```python
from build123d import *

# Parameters (mm, degrees)
BOSS_EXTRUDE1_DEPTH       = 276.125
SKETCH3_W                 = 268.125
SKETCH3_H                 = 78.2
CUT_EXTRUDE1_DEPTH        = 21
SKETCH4_W                 = 14
SKETCH4_H                 = 14.4
CUT_EXTRUDE2_DEPTH        = 4
FILLET1_R                 = 5
FILLET4_R                 = 3
FILLET5_R                 = 4
FILLET6_R                 = 4
SKETCH5_R                 = 2.5
BOSS_EXTRUDE2_DEPTH       = 5
FILLET7_R                 = 3
M2X0_4_TAPPED_HOLE4_D     = 1.6
M2X0_4_TAPPED_HOLE4_DEPTH = 3.719311505
M2X0_4_TAPPED_HOLE4_TIP   = 0.480688495
CUT_EXTRUDE3_DEPTH        = 2
FILLET8_R                 = 3
SKETCH10_R                = 5
CUT_EXTRUDE4_DEPTH        = 0.5


with BuildPart() as part:
    # Sketch1 → Boss-Extrude1 (new body)
    with BuildSketch(Plane(origin=(0, 0, 0), x_dir=(0, 0, -1), z_dir=(1, 0, 0))):
        Polygon((43.1, -11), (43.1, -18.54), (-43.1, -11), (-43.1, 11), (43.1, 11), align=None)
    extrude(amount=BOSS_EXTRUDE1_DEPTH)

    # Sketch3 → Cut-Extrude1 (cut)
    with BuildSketch(Plane(origin=(0, 11, 0), x_dir=(1, 0, 0), z_dir=(0, 1, 0))):
        with Locations((138.0625, 0)):
            Rectangle(SKETCH3_W, SKETCH3_H)
    extrude(amount=-CUT_EXTRUDE1_DEPTH, mode=Mode.SUBTRACT)

    # Sketch4 → Cut-Extrude2 (cut)
    with BuildSketch(Plane.XY.offset(-39.1)):
        with Locations((257.755, 3.8)):
            Rectangle(SKETCH4_W, SKETCH4_H)
    extrude(amount=-CUT_EXTRUDE2_DEPTH, mode=Mode.SUBTRACT)

    # Fillet1
    fillet1_edges = [part.edges().sort_by_distance(p)[0] for p in [
        (276.125, -3.77, -43.1),
        (276.125, 0, 43.1),
        (0, -3.77, -43.1),
        (0, 0, 43.1),
    ]]
    fillet(fillet1_edges, radius=FILLET1_R)

    # Fillet4
    fillet4_edges = [part.edges().sort_by_distance(p)[0] for p in [
        (272.125, 0.5, -39.1),
        (272.125, 0.5, 39.1),
        (4, 0.5, 39.1),
        (4, 0.5, -39.1),
    ]]
    fillet(fillet4_edges, radius=FILLET4_R)

    # Fillet5
    fillet5_edges = [part.edges().sort_by_distance(p)[0] for p in [
        (264.755, 11, -41.1),
        (264.755, -3.4, -41.1),
        (250.755, -3.4, -41.1),
        (250.755, 11, -41.1),
    ]]
    fillet(fillet5_edges, radius=FILLET5_R)

    # Fillet6
    fillet6_edges = [part.edges().sort_by_distance(p)[0] for p in [
        (274.660533906, 11, 41.635533906),
        (276.125, 11, 0),
        (274.660533906, 11, -41.635533906),
        (269.94, 11, -43.1),
        (265.926572875, 9.828427125, -43.1),
        (264.755, 3.8, -43.1),
        (263.583427125, -2.228427125, -43.1),
        (257.755, -3.4, -43.1),
        (251.926572875, -2.228427125, -43.1),
        (250.755, 3.8, -43.1),
        (249.583427125, 9.828427125, -43.1),
        (125.8775, 11, -43.1),
        (1.464466094, 11, -41.635533906),
        (0, 11, 0),
        (1.464466094, 11, 41.635533906),
        (138.0625, 11, 43.1),
    ]]
    fillet(fillet6_edges, radius=FILLET6_R - 0.0001)  # a hair under: the kernel refuses the full size

    # Sketch5 → Boss-Extrude2 (add)
    with BuildSketch(Plane(origin=(0, -10, 0), x_dir=(1, 0, 0), z_dir=(0, 1, 0))):
        with Locations(Location((240.4, 19.1, 0), (0, 0, 90))):
            Circle(SKETCH5_R)
        with Locations(Location((240.4, -19, 0), (0, 0, 90))):
            Circle(SKETCH5_R)
        with BuildLine():
            Line((9.8, 21.6), (4, 21.6))
            Line((4, 21.6), (4, 16.6))
            Line((4, 16.6), (9.8, 16.6))
            ThreePointArc((9.8, 16.6), (12.3, 19.1), (9.8, 21.6))
        make_face()
        with BuildLine():
            Line((9.8, -16.5), (4, -16.5))
            Line((4, -16.5), (4, -21.5))
            Line((4, -21.5), (9.8, -21.5))
            ThreePointArc((9.8, -21.5), (12.3, -19), (9.8, -16.5))
        make_face()
        with BuildLine():
            Line((244.225, 35.5), (244.225, 39.1))
            Line((244.225, 39.1), (249.225, 39.1))
            Line((249.225, 39.1), (249.225, 35.5))
            ThreePointArc((249.225, 35.5), (246.725, 33), (244.225, 35.5))
        make_face()
        with BuildLine():
            Line((265.995, 35.5), (265.995, 39.1))
            Line((265.995, 39.1), (269.125, 39.1))
            ThreePointArc((269.125, 39.1), (271.246320344, 38.221320344), (272.125, 36.1))
            Line((272.125, 36.1), (272.125, 33))
            Line((272.125, 33), (268.495, 33))
            ThreePointArc((268.495, 33), (266.727233047, 33.732233047), (265.995, 35.5))
        make_face()
        with BuildLine():
            Line((249.225, -35.5), (249.225, -39.1))
            Line((249.225, -39.1), (244.225, -39.1))
            Line((244.225, -39.1), (244.225, -35.5))
            ThreePointArc((244.225, -35.5), (246.725, -33), (249.225, -35.5))
        make_face()
        with BuildLine():
            Line((268.495, -33), (272.125, -33))
            Line((272.125, -33), (272.125, -36.1))
            ThreePointArc((272.125, -36.1), (271.246320344, -38.221320344), (269.125, -39.1))
            Line((269.125, -39.1), (265.995, -39.1))
            Line((265.995, -39.1), (265.995, -35.5))
            ThreePointArc((265.995, -35.5), (266.727233047, -33.732233047), (268.495, -33))
        make_face()
    extrude(amount=BOSS_EXTRUDE2_DEPTH)

    # Fillet7
    fillet7_edges = [part.edges().sort_by_distance(p)[0] for p in [
        (4, -7.5, 16.5),
        (4, -7.5, 21.5),
        (244.225, -7.5, 39.1),
        (249.225, -7.5, 39.1),
        (265.995, -7.5, 39.1),
        (272.125, -7.5, 33),
        (249.225, -7.5, -39.1),
        (244.225, -7.5, -39.1),
        (4, -7.5, -21.6),
        (4, -7.5, -16.6),
        (272.125, -7.5, -33),
        (265.995, -7.5, -39.1),
    ]]
    fillet(fillet7_edges, radius=FILLET7_R)

    # M2x0.4 Tapped Hole4
    with Locations(Plane(origin=(0, -5, 0), x_dir=(1, 0, 0), z_dir=(0, 1, 0))):
        with Locations((9.8, 19.1), (9.8, -19), (240.4, 19.1), (240.4, -19), (246.725, 35.5), (268.495, 35.5), (268.495, -35.5), (246.725, -35.5)):
            Hole(M2X0_4_TAPPED_HOLE4_D / 2, depth=M2X0_4_TAPPED_HOLE4_DEPTH)
            with Locations((0, 0, -(M2X0_4_TAPPED_HOLE4_DEPTH + M2X0_4_TAPPED_HOLE4_TIP / 2))):  # 118° drill point
                Cone(0, M2X0_4_TAPPED_HOLE4_D / 2, M2X0_4_TAPPED_HOLE4_TIP, mode=Mode.SUBTRACT)

    # Sketch9 → Cut-Extrude3 (cut)
    with BuildSketch(Plane(origin=(0, -10, 0), x_dir=(1, 0, 0), z_dir=(0, 1, 0))):
        Polygon((243.575047285, -10.7), (253.575047285, -10.7), (253.575047285, -0.7), (243.575047285, -0.7), (225.575047285, -0.7), (225.575047285, 25.3), (171.075047285, 25.3), (171.075047285, -10.7), align=None)
    extrude(amount=-CUT_EXTRUDE3_DEPTH, mode=Mode.SUBTRACT)

    # Fillet8
    fillet8_edges = [part.edges().sort_by_distance(p)[0] for p in [
        (253.575047285, -11, 0.7),
        (253.575047285, -11, 10.7),
        (171.075047285, -11, 10.7),
        (171.075047285, -11, -25.3),
        (225.575047285, -11, -25.3),
    ]]
    fillet(fillet8_edges, radius=FILLET8_R)

    # Sketch10 → Cut-Extrude4 (cut)
    with BuildSketch(Plane(origin=(0, -14.657850216, 1.282136782), x_dir=(1, 0, 0), z_dir=(0, -0.9961962259253339, 0.08713827776655463))):
        with Locations(Location((266.125, -34.551601007, 0), (0, 0, 270))):
            Circle(SKETCH10_R)
        with Locations(Location((266.125, 31.977536282, 0), (0, 0, 270))):
            Circle(SKETCH10_R)
        with Locations(Location((10, 31.977536282, 0), (0, 0, 270))):
            Circle(SKETCH10_R)
        with Locations(Location((10, -34.551601007, 0), (0, 0, 270))):
            Circle(SKETCH10_R)
    extrude(amount=-CUT_EXTRUDE4_DEPTH, mode=Mode.SUBTRACT)


solid = part.part
```
The model under review builds one solid part; all positions refer to its coordinate system, in mm. A direction names the side the tool comes from. Round coordinates to 2 decimals unless told otherwise and drop trailing zeros. Use a Markdown table: item, result.
Q1. Mouldability with a two-part tool opening along Y and no side actions: class faces 3 (the cylindrical face through (12.3, -7.5, -19)), 4 (the cylindrical face through (14.957, -17.366, -32.511)), 5 (the cylindrical face through (271.082, -17.366, -32.511)), 6 (the flat face through (240, -5, 20)) as +Y half, -Y half, draft (parallel to the pull), parting line (faces both ways), or undercut.
Values:
| item | result |
|---|---|
| face 3 | draft |
| face 4 | undercut |
| face 5 | undercut |
| face 6 | +Y half |
Q2. Tool access review of faces 1 (the flat face through (136, -10, -1)), 2 (the flat face through (136.13, -14.823, -0.603)): name each direction out of +Z, -Z, +X, -X, +Y, -Y from which nothing blocks a thin tool from reaching the whole face with its end or side.
Values:
| item | result |
|---|---|
| face 1 | +Y |
| face 2 | +Z, +X, -X, -Y |
Q3. Clearance check with flat-ended pins moving along their axes: P1, Ø1.8, axis at x = 246.725, z = -35.5, coming from the +Y side; P2, Ø3, axis at x = 49.5, z = 19, coming from the +Y side. State where each tip first meets the part, or that it passes through.
Values:
| item | result |
|---|---|
| P1 | stops at y = -5 |
| P2 | stops at y = -10 |
Q4. For line 1 (X direction, y = -7.05, z = -35.5) (3 decimals); line 2 (Z direction, x = 240.4, y = -6.1); line 3 (Z direction, x = 241.5, y = -0.75), list the stretches that pass through material, from the lowest coordinate up.
Values:
| item | result |
|---|---|
| line 1 | x = 0 to 4, 244.225 to 245.925, 247.525 to 249.225, 265.995 to 267.695, 269.295 to 276.125 |
| line 2 | z = -43.1 to -39.1, -21.6 to -19.9, -18.3 to -16.6, 16.5 to 18.2, 19.8 to 21.5, 39.1 to 43.1 |
| line 3 | z = -43.1 to -39.1, 39.1 to 43.1 |
